```python
from build123d import *

# Parameters (mm, degrees)
F1_DEPTH  = 7
F4_R      = 27.5
F3_R      = 25
F7_R      = 25
F9_DEPTH  = 5
F10_DEPTH = 24.4
F11_DEPTH = 8
F14_DEPTH = 48.7
F15_DEPTH = 60.7407367097
F12_R     = 3.5
F16_DEPTH = 12
F17_R     = 3
F18_DEPTH = 12


with BuildPart() as f1:
    # F0 (on Front) → F1 (new body, symmetric)
    with BuildSketch(Plane.XZ):
        with BuildLine():
            ThreePointArc((-10, 56), (-7.0710678119, 48.9289321881), (0, 46))
            ThreePointArc((0, 46), (7.0710678119, 48.9289321881), (10, 56))
            ThreePointArc((10, 56), (0, 66), (-10, 56))
        make_face()
        with BuildLine():
            ThreePointArc((4, 56), (2.8284271247, 53.1715728753), (0, 52))
            ThreePointArc((0, 52), (-2.8284271247, 58.8284271247), (4, 56))
        make_face(mode=Mode.SUBTRACT)
    extrude(amount=F1_DEPTH, both=True)



with BuildPart() as f5:
    # F4 (on Front) → F5 section 0
    with BuildSketch(Plane.XZ):
        Circle(F4_R)
    # F3 (on offset) → F5 section 1
    with BuildSketch(Plane.XZ.offset(10)):
        Circle(F3_R)
    loft()

    # F4 (on Front) → F8 section 0
    with BuildSketch(Plane.XZ):
        Circle(F4_R)
    # F7 (on offset) → F8 section 1
    with BuildSketch(Plane.XZ.offset(-10)):
        Circle(F7_R)
    loft()


with BuildPart() as f1_1:
    add(f1.part)

    add(f5.part)  # F9 merges F5
    # F0 (on Front) → F9 (join, symmetric)
    with BuildSketch(Plane.XZ):
        with BuildLine():
            Line((0, 46), (0, 27.5))
            ThreePointArc((0, 27.5), (5.0878352391, 27.0252462076), (10, 25.6173769149))
            Line((10, 25.6173769149), (10, 56))
            ThreePointArc((10, 56), (7.0710678119, 48.9289321881), (0, 46))
        make_face()
        with BuildLine():
            ThreePointArc((-10, 25.6173769149), (-5.0878352391, 27.0252462076), (0, 27.5))
            Line((0, 27.5), (0, 46))
            ThreePointArc((0, 46), (-7.0710678119, 48.9289321881), (-10, 56))
            Line((-10, 56), (-10, 25.6173769149))
        make_face()
        with BuildLine():
            ThreePointArc((-10, 22.9128784748), (-5.1077410922, 24.4726578233), (0, 25))
            Line((0, 25), (0, 27.5))
            ThreePointArc((0, 27.5), (-5.0878352391, 27.0252462076), (-10, 25.6173769149))
            Line((-10, 25.6173769149), (-10, 22.9128784748))
        make_face()
        with BuildLine():
            Line((0, 27.5), (0, 25))
            ThreePointArc((0, 25), (5.1077410922, 24.4726578233), (10, 22.9128784748))
            Line((10, 22.9128784748), (10, 25.6173769149))
            ThreePointArc((10, 25.6173769149), (5.0878352391, 27.0252462076), (0, 27.5))
        make_face()
    extrude(amount=F9_DEPTH, both=True)

    # F0 (on Front) → F10 (cut, symmetric)
    with BuildSketch(Plane.XZ):
        with BuildLine():
            Line((0, 0), (0, 20))
            ThreePointArc((0, 20), (-20, 0), (0, -20))
            Line((0, -20), (0, 0))
        make_face()
        with BuildLine():
            ThreePointArc((0, -20), (14.1421356237, -14.1421356237), (20, 0))
            ThreePointArc((20, 0), (14.1421356237, 14.1421356237), (0, 20))
            Line((0, 20), (0, 0))
            Line((0, 0), (0, -20))
        make_face()
    extrude(amount=F10_DEPTH, both=True, mode=Mode.SUBTRACT)

    # F0 (on Front) → F11 (join, symmetric)
    with BuildSketch(Plane.XZ):
        with BuildLine():
            Line((49.5512701892, -14.1746824527), (27.4632034356, -1.4221311666))
            ThreePointArc((27.4632034356, -1.4221311666), (26.5074954683, -7.3213853878), (24.2999474789, -12.8748806799))
            Line((24.2999474789, -12.8748806799), (43.8012701892, -24.1339745962))
            Line((43.8012701892, -24.1339745962), (49.5512701892, -14.1746824527))
        make_face()
        Polygon((56.4794734195, -18.1746824527), (49.5512701892, -14.1746824527), (43.8012701892, -24.1339745962), (50.7294734195, -28.1339745962), align=None)
        Polygon((42.8012701892, -25.8660254038), (37.0512701892, -35.8253175473), (43.9794734195, -39.8253175473), (49.7294734195, -29.8660254038), align=None)
        with BuildLine():
            ThreePointArc((23.2999474789, -14.6069314874), (19.5942534709, -19.2954717724), (14.9632034356, -23.0727662612))
            Line((14.9632034356, -23.0727662612), (37.0512701892, -35.8253175473))
            Line((37.0512701892, -35.8253175473), (42.8012701892, -25.8660254038))
            Line((42.8012701892, -25.8660254038), (23.2999474789, -14.6069314874))
        make_face()
        with BuildLine():
            Line((27.4632034356, -1.4221311666), (25, 0))
            ThreePointArc((25, 0), (24.2727490338, -5.9861218113), (22.1333076528, -11.623970593))
            Line((22.1333076528, -11.623970593), (24.2999474789, -12.8748806799))
            ThreePointArc((24.2999474789, -12.8748806799), (26.5074954683, -7.3213853878), (27.4632034356, -1.4221311666))
        make_face()
        with BuildLine():
            ThreePointArc((21.1333076528, -13.3560214006), (17.3205080757, -18.0277563773), (12.5, -21.6506350946))
            Line((12.5, -21.6506350946), (14.9632034356, -23.0727662612))
            ThreePointArc((14.9632034356, -23.0727662612), (19.5942534709, -19.2954717724), (23.2999474789, -14.6069314874))
            Line((23.2999474789, -14.6069314874), (21.1333076528, -13.3560214006))
        make_face()
    extrude(amount=F11_DEPTH, both=True)

    # F13 (on face) → F14 (cut)
    with BuildSketch(Plane(origin=(50.2294734195, 0, -29), x_dir=(0, 1, 0), z_dir=(0.8660254038, 0, -0.5))):
        Polygon((16.3611844182, 1), (8, 1), (-8, 1), (-11.9865061715, 1), (-11.9865061715, -1), (-8, -1), (8, -1), (16.3611844182, -1), align=None)
    extrude(amount=-F14_DEPTH, mode=Mode.SUBTRACT)

    # F12 (on face) → F15 (cut, through all)
    with BuildSketch(Plane(origin=(6.25, 0, 10.8253175473), x_dir=(0.8660254038, 0, -0.5), z_dir=(0.5, 0, 0.8660254038))):
        with BuildLine():
            ThreePointArc((58, 0), (55.6568542495, -5.6568542495), (50, -8))
            Line((50, -8), (58, -8))
            Line((58, -8), (58, 0))
        make_face()
        with BuildLine():
            Line((58, 8), (50, 8))
            ThreePointArc((50, 8), (55.6568542495, 5.6568542495), (58, 0))
            Line((58, 0), (58, 8))
        make_face()
    extrude(amount=-F15_DEPTH, mode=Mode.SUBTRACT)

    # F12 (on face) → F16 (cut)
    with BuildSketch(Plane(origin=(6.25, 0, 10.8253175473), x_dir=(0.8660254038, 0, -0.5), z_dir=(0.5, 0, 0.8660254038))):
        with Locations((50, 0)):
            Circle(F12_R)
    extrude(amount=-F16_DEPTH, mode=Mode.SUBTRACT)

    # F17 (on face) → F18 (cut)
    with BuildSketch(Plane(origin=(-6.25, 0, -10.8253175473), x_dir=(0.8660254038, 0, -0.5), z_dir=(-0.5, 0, -0.8660254038))):
        with Locations((50, 0)):
            Circle(F17_R)
    extrude(amount=-F18_DEPTH, mode=Mode.SUBTRACT)


solid = f1_1.part
```
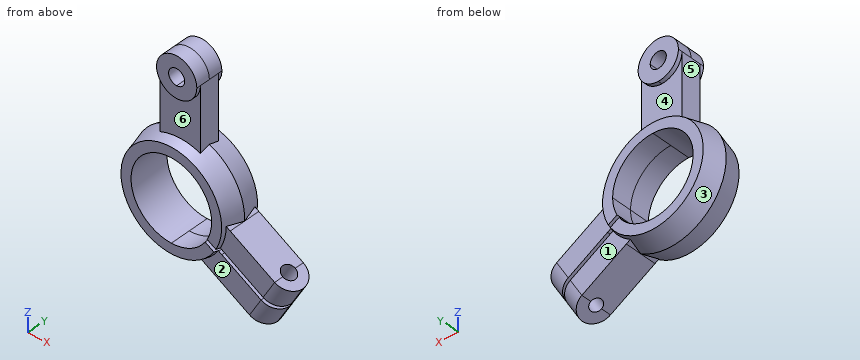
For this review, take the finished solid that the model builds, in its own axes (mm). Face numbers are marked on the shaded views. A direction names the side the tool comes from. Give positions to 0.01 mm unless a question says otherwise; leave off trailing zeros. Write each loop counter-clockwise with the first axis right and the second up, starting at its lowest first coordinate (ties: lowest second). Pieces come first, ordered by that corner, then holes.
Item 1: The part is to be moulded in two halves that separate along Z. For the marked faces 4, 5 and 6, say which applies: +Z half, -Z half, draft (parallel to the pull), parting line (faces both ways), or undercut.
Item 2: Insertion check: P1, Ø10, axis at x = 45, z = -19.5, coming from the +Y side; P2, Ø8, axis at y = -0.5, z = 42.5, coming from the -X side; P3, Ø19, axis at x = 34.5, z = -8, coming from the -Y side; P4, Ø12, axis at x = -10.5, z = -7, coming from the -Y side. Each pin has a flat end and moves straight along its axis. Give the tip position at first contact, or say it passes through.
Item 3: Take a section at A-A (z = 35). Give the boundary of the cut face in (x, y), and give its area (3 significant figures).
Item 4: Wall thickness on probe 1 along X at (y, z) = (4.5, 56); probe 2 along Z at (x, y) = (18.5, 9); probe 3 along X at (y, z) = (-5, -12.5): over which ranges is each line inside the solid? List them lowest first.
Item 5: Machinability: for the marked faces 1, 2 and 3, which of the approach directions +Z, -Z, +X, -X, +Y, -Y give a long, thin tool a straight path to every point of the face, cutting with its end or side? Answer none if there is none.
Established:
1. face 4: undercut
1. face 5: draft
1. face 6: undercut
2. P1: stops at y = 8
2. P2: stops at x = -10
2. P3: stops at y = -8
2. P4: passes through
3. outline: (-10, -5) - (10, -5) - (10, 5) - (-10, 5) - close
3. area: 200 mm2
4. probe 1: x = -10 to -4, 4 to 10
4. probe 2: z = -17.18 to -11.84, -9.53 to -7.6, 7.6 to 17.18
4. probe 3: x = -23.08 to -15.61, 15.61 to 19.65, 23.65 to 46.65
5. face 1: -Z, +X, +Y
5. face 2: -Z, +X, -Y
5. face 3: +Y
